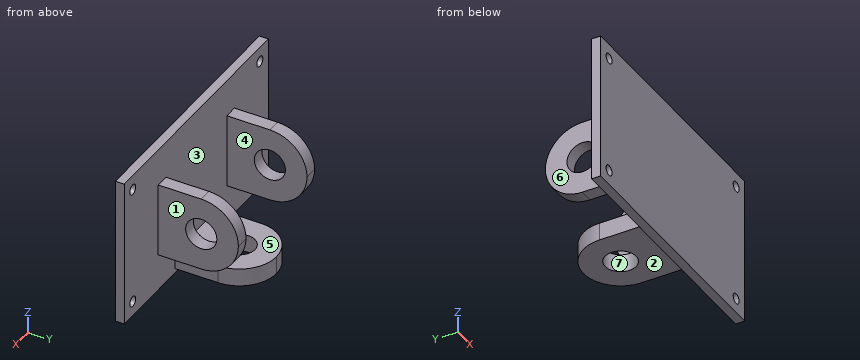
from build123d import *

# Parameters (mm, degrees)
SKICA1_W                          = 85
SKICA1_H                          = 50
P_IDAT_VYSUNUT_M1_DEPTH           = 3
SKICA2_W                          = 4.5
SKICA2_H                          = 25
SKICA2_W_2                        = 25
SKICA2_H_2                        = 6
P_IDAT_VYSUNUT_M2_DEPTH           = 27
ZAOBLIT1_R                        = 12.5
SKICA3_R                          = 5.25
ODEBRAT_VYSUNUT_M1_DEPTH          = 76.828754441
SKICA4_R                          = 5.25
ODEBRAT_VYSUNUT_M2_DEPTH          = 68.175144213
D_RY_PRO_KOL_K_VELIKOST_MM1_D     = 3.5
D_RY_PRO_KOL_K_VELIKOST_MM1_DEPTH = 10
D_RY_PRO_KOL_K_VELIKOST_MM1_TIP   = 1.051506083


with BuildPart() as part:
    # Skica1 → Přidat vysunutím1 (new body)
    with BuildSketch(Plane(origin=(0, 0, 0), x_dir=(1, 0, 0), z_dir=(0, 1, 0))):
        Rectangle(SKICA1_W, SKICA1_H)
    extrude(amount=P_IDAT_VYSUNUT_M1_DEPTH)

    # Skica2 → Přidat vysunutím2 (add)
    with BuildSketch(Plane(origin=(0, 3, 0), x_dir=(1, 0, 0), z_dir=(0, 1, 0))):
        with Locations((-20.25, 0)):
            Rectangle(SKICA2_W, SKICA2_H)
        with Locations((0, 20.5)):
            Rectangle(SKICA2_W_2, SKICA2_H_2)
        with Locations((20.25, 0)):
            Rectangle(SKICA2_W, SKICA2_H)
    extrude(amount=P_IDAT_VYSUNUT_M2_DEPTH)

    # Zaoblit1
    zaoblit1_edges = [part.edges().sort_by_distance(p)[0] for p in [
        (-20.25, 30, -12.5),
        (-20.25, 30, 12.5),
        (-12.5, 30, -20.5),
        (12.5, 30, -20.5),
        (20.25, 30, -12.5),
        (20.25, 30, 12.5),
    ]]
    fillet(zaoblit1_edges, radius=ZAOBLIT1_R - 0.0001)  # a hair under: the kernel refuses the full size

    # Skica3 → Odebrat vysunutím1 (cut, through all)
    with BuildSketch(Plane.ZY.offset(22.5)):
        with Locations((0, 17.5)):
            Circle(SKICA3_R)
    extrude(amount=-ODEBRAT_VYSUNUT_M1_DEPTH, mode=Mode.SUBTRACT)

    # Skica4 → Odebrat vysunutím2 (cut, through all)
    with BuildSketch(Plane.XY.offset(-17.5)):
        with Locations((0, 17.5)):
            Circle(SKICA4_R)
    extrude(amount=-ODEBRAT_VYSUNUT_M2_DEPTH, mode=Mode.SUBTRACT)

    # Díry pro kolík, velikost mm1
    with Locations(Plane(origin=(0, 3, 0), x_dir=(1, 0, 0), z_dir=(0, 1, 0))):
        with Locations((-37.5, 20), (37.5, 20), (37.5, -20), (-37.5, -20)):
            Hole(D_RY_PRO_KOL_K_VELIKOST_MM1_D / 2, depth=D_RY_PRO_KOL_K_VELIKOST_MM1_DEPTH)
            with Locations((0, 0, -(D_RY_PRO_KOL_K_VELIKOST_MM1_DEPTH + D_RY_PRO_KOL_K_VELIKOST_MM1_TIP / 2))):  # 118° drill point
                Cone(0, D_RY_PRO_KOL_K_VELIKOST_MM1_D / 2, D_RY_PRO_KOL_K_VELIKOST_MM1_TIP, mode=Mode.SUBTRACT)


solid = part.part
Input: part model. Units: mm. Frame: model coordinates. Face numbers are marked on the shaded views. A direction names the side the tool comes from. Give positions to 0.01 mm unless a question says otherwise; leave off trailing zeros. Order: outer loops, then holes, each group sorted by start corner. A loop starts at its lowest first (then second) coordinate and runs counter-clockwise, first axis right, second up. Notation, with made-up numbers: (39, 78) - (47, 78) arc R29 ccw to (47, 102) - close; hole circle Ø6 at (-12, 64). An arc over 180 degrees is marked (long way). Answer as a JSON object with one key per item and string values. Group by question number.
Q1. Cut plane D-D, the plane x = -9. Output: boundary loops of the cut face in (y, z), then the cut area to 3 significant figures.
Q2. Cut plane C-C, the plane x = 3. Output: boundary loops of the cut face in (y, z), then the cut area to 3 significant figures.
Q3. Cut plane B-B, the plane y = 28. Output: boundary loops of the cut face in (x, z), then the cut area to 3 significant figures.
Q4. First-contact query: pin 1 Ø6 at (y, z) = (20.5, -9) entering from +X; pin 2 Ø3 at (x, z) = (-37.5, 20) entering from -Y; pin 3 Ø3 at (y, z) = (7, -22) entering from -X; pin 4 Ø2 at (x, y) = (20, 8) entering from +Z. Flat tips, straight axial feed; report the tip coordinate or a pass-through.
Q5. Set-up query: the marked faces 5, 6 and 7. Return all of +Z, -Z, +X, -X, +Y, -Y with unobstructed straight access to the full face (end or side cutting, diameter ignored); none if empty.
Q6. Cut plane A-A, the plane z = 20. Output: boundary loops of the cut face in (x, y).
Q7. Line query: probe 1 along X at (y, z) = (11.5, 0); probe 2 along X at (y, z) = (1.8, -20); probe 3 along Z at (x, y) = (-37, 1). Output: solid intervals per line, ascending.
Q8. Mould query, pull axis X, two halves, no side actions, for the marked faces 1, 2, 3 and 4. Classes: pulls with the +X half, pulls with the -X half, needs draft (parallel to the pull), parting line crosses it, or undercut.
Results:
{
 "1": {"outline": "(0, -25) - (3, -25) - (3, -23.5) - (26.17, -23.5) - (26.17, -17.5) - (3, -17.5) - (3, 25) - (0, 25) - close", "area": "289 mm^2"},
 "2": {"outline": "(0, -25) - (3, -25) - (3, -23.5) - (13.19, -23.5) - (13.19, -17.5) - (3, -17.5) - (3, 25) - (0, 25) - close; (21.81, -23.5) - (29.63, -23.5) - (29.63, -17.5) - (21.81, -17.5) - close", "area": "258 mm^2"},
 "3": {"outline": "(-22.5, -6.78) - (-18, -6.78) - (-18, 6.78) - (-22.5, 6.78) - close; (-6.78, -23.5) - (6.78, -23.5) - (6.78, -17.5) - (-6.78, -17.5) - close; (18, -6.78) - (22.5, -6.78) - (22.5, 6.78) - (18, 6.78) - close", "area": "203 mm^2"},
 "4": {"pin 1": "x = 22.5", "pin 2": "through", "pin 3": "x = -12.5", "pin 4": "z = 12.5"},
 "5": {"face 5": "+Z, +X, -X, +Y", "face 6": "+Z, -Z, -X, +Y", "face 7": "+Z, -Z"},
 "6": {"outline": "(-42.5, 0) - (-39.25, 0) - (-39.25, 3) - (-42.5, 3) - close; (-35.75, 0) - (35.75, 0) - (35.75, 3) - (-35.75, 3) - close; (39.25, 0) - (42.5, 0) - (42.5, 3) - (39.25, 3) - close"},
 "7": {"probe 1": "-22.5 to -18, 18 to 22.5", "probe 2": "-42.5 to -39.25, -35.75 to 35.75, 39.25 to 42.5", "probe 3": "-25 to -21.68, -18.32 to 18.32, 21.68 to 25"},
 "8": {"face 1": "pulls with the +X half", "face 2": "needs draft", "face 3": "undercut", "face 4": "undercut"}
}
